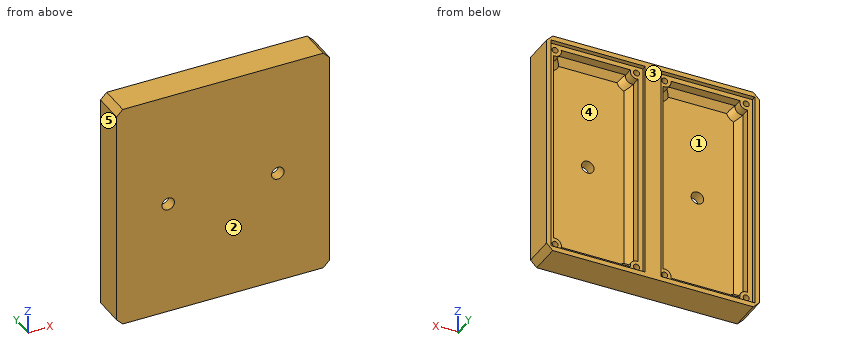
from build123d import *

# Parameters (mm, degrees)
SKETCH2_W           = 68
SKETCH2_H           = 73
SKETCH2_W_2         = 30
SKETCH2_H_2         = 70
BOSS_EXTRUDE1_DEPTH = 10
SKETCH2_3_W         = 30
SKETCH2_3_H         = 70
CUT_EXTRUDE2_DEPTH  = 1.5
SKETCH3_W           = 27
SKETCH3_H           = 67
CUT_EXTRUDE3_DEPTH  = 5
SKETCH4_R           = 2
BOSS_EXTRUDE2_DEPTH = 5
CUT_EXTRUDE4_START  = -5
SKETCH5_R           = 0.95
CUT_EXTRUDE4_DEPTH  = 5
CHAMFER1_SIZE       = 2
CHAMFER2_SIZE       = 2
SKETCH6_R           = 2
CUT_EXTRUDE5_DEPTH  = 4


with BuildPart() as part:
    # Sketch2 → Boss-Extrude1 (new body)
    # profile 1 of 3: a face of its own
    with BuildSketch(Plane(origin=(0, 0, 0), x_dir=(1, 0, 0), z_dir=(0, 1, 0))):
        Rectangle(SKETCH2_W, SKETCH2_H)
        with Locations((17.5, 0)):
            Rectangle(SKETCH2_W_2, SKETCH2_H_2, mode=Mode.SUBTRACT)
        with Locations((-17.5, 0)):
            Rectangle(SKETCH2_W_2, SKETCH2_H_2, mode=Mode.SUBTRACT)
    # profile 2 of 3: a face of its own
    with BuildSketch(Plane(origin=(0, 0, 0), x_dir=(1, 0, 0), z_dir=(0, 1, 0))):
        with Locations((17.5, 0)):
            Rectangle(SKETCH2_W_2, SKETCH2_H_2)
    # profile 3 of 3: a face of its own
    with BuildSketch(Plane(origin=(0, 0, 0), x_dir=(1, 0, 0), z_dir=(0, 1, 0))):
        with Locations((-17.5, 0)):
            Rectangle(SKETCH2_W_2, SKETCH2_H_2)
    extrude(amount=-BOSS_EXTRUDE1_DEPTH)

    # Sketch2<3> → Cut-Extrude2 (cut)
    with BuildSketch(Plane(origin=(0, 0, 0), x_dir=(1, 0, 0), z_dir=(0, 1, 0))):
        with Locations((-17.5, 0)):
            Rectangle(SKETCH2_3_W, SKETCH2_3_H)
        with Locations((17.5, 0)):
            Rectangle(SKETCH2_3_W, SKETCH2_3_H)
    extrude(amount=-CUT_EXTRUDE2_DEPTH, mode=Mode.SUBTRACT)

    # Sketch3 → Cut-Extrude3 (cut)
    with BuildSketch(Plane(origin=(0, -1.5, 0), x_dir=(1, 0, 0), z_dir=(0, 1, 0))):
        with Locations((-17.5, 0)):
            Rectangle(SKETCH3_W, SKETCH3_H)
        with Locations((17.5, 0)):
            Rectangle(SKETCH3_W, SKETCH3_H)
    extrude(amount=-CUT_EXTRUDE3_DEPTH, mode=Mode.SUBTRACT)

    # Sketch4 → Boss-Extrude2 (add)
    with BuildSketch(Plane(origin=(0, -6.5, 0), x_dir=(1, 0, 0), z_dir=(0, 1, 0))):
        with Locations((-30.5, 33)):
            Circle(SKETCH4_R)
        with Locations((-4.5, 33)):
            Circle(SKETCH4_R)
        with Locations((-4.5, -33)):
            Circle(SKETCH4_R)
        with Locations((-30.5, -33)):
            Circle(SKETCH4_R)
        with Locations((30.5, -33)):
            Circle(SKETCH4_R)
        with Locations((4.5, -33)):
            Circle(SKETCH4_R)
        with Locations((4.5, 33)):
            Circle(SKETCH4_R)
        with Locations((30.5, 33)):
            Circle(SKETCH4_R)
    extrude(amount=BOSS_EXTRUDE2_DEPTH)

    # Sketch5 → Cut-Extrude4 (cut)
    with BuildSketch(Plane(origin=(0, -1.5, 0), x_dir=(1, 0, 0), z_dir=(0, 1, 0)).offset(CUT_EXTRUDE4_START)):
        with Locations(Location((-30.5, 33, 0), (0, 0, 270))):
            Circle(SKETCH5_R)
        with Locations(Location((-4.5, 33, 0), (0, 0, 270))):
            Circle(SKETCH5_R)
        with Locations(Location((-4.5, -33, 0), (0, 0, 270))):
            Circle(SKETCH5_R)
        with Locations(Location((-30.5, -33, 0), (0, 0, 270))):
            Circle(SKETCH5_R)
        with Locations(Location((30.5, -33, 0), (0, 0, 270))):
            Circle(SKETCH5_R)
        with Locations(Location((4.5, -33, 0), (0, 0, 270))):
            Circle(SKETCH5_R)
        with Locations(Location((4.5, 33, 0), (0, 0, 270))):
            Circle(SKETCH5_R)
        with Locations(Location((30.5, 33, 0), (0, 0, 270))):
            Circle(SKETCH5_R)
    extrude(amount=CUT_EXTRUDE4_DEPTH, mode=Mode.SUBTRACT)

    # Chamfer1
    chamfer1_edges = [part.edges().sort_by_distance(p)[0] for p in [
        (-34, -5, 36.5),
        (-34, -5, -36.5),
        (34, -5, -36.5),
        (34, -5, 36.5),
    ]]
    chamfer(chamfer1_edges, length=CHAMFER1_SIZE)

    # Chamfer2
    chamfer2_edges = [part.edges().sort_by_distance(p)[0] for p in [
        (-4, -6.5, 0),
        (-5.914213562, -6.5, 31.585786438),
        (-17.5, -6.5, 33.5),
        (-29.085786438, -6.5, 31.585786438),
        (31, -6.5, 0),
        (29.085786438, -6.5, 31.585786438),
        (17.5, -6.5, 33.5),
        (5.914213562, -6.5, 31.585786438),
        (4, -6.5, 0),
        (5.914213562, -6.5, -31.585786438),
        (17.5, -6.5, -33.5),
        (29.085786438, -6.5, -31.585786438),
        (-31, -6.5, 0),
        (-29.085786438, -6.5, -31.585786438),
        (-17.5, -6.5, -33.5),
        (-5.914213562, -6.5, -31.585786438),
    ]]
    chamfer(chamfer2_edges, length=CHAMFER2_SIZE)

    # Sketch6 → Cut-Extrude5 (cut)
    with BuildSketch(Plane.XZ.offset(10)):
        with Locations(Location((-17.5, 0, 0), (0, 0, 270))):
            Circle(SKETCH6_R)
        with Locations(Location((17.5, 0, 0), (0, 0, 270))):
            Circle(SKETCH6_R)
    extrude(amount=-CUT_EXTRUDE5_DEPTH, mode=Mode.SUBTRACT)


solid = part.part
Verification items for the finished model (mm, model axes). Face numbers are marked on the shaded views. A direction names the side the tool comes from. Round coordinates to 2 decimals unless told otherwise and drop trailing zeros. Loops run counter-clockwise (first coordinate to the right, second up) from the corner with the lowest first, then second, coordinate; pieces in that order, holes last. Notation, with made-up numbers: (-14, 65.5) - (33, 65.5) arc R16 cw to (33, 88.5) - close; hole circle Ø9 at (-37, -21). An arc over 180 degrees is marked (long way). Use a Markdown table: item, result. Add a question column.
1. Section check C-C, the plane z = 13.5. Record the boundary of the cut face in (x, y).
2. Thickness scan on probe 1 along X at (y, z) = (-9.25, 0); probe 2 along X at (y, z) = (-1, 17); probe 3 along X at (y, z) = (-5.25, 33). Record the ranges inside material, lowest first. Write a range as [from, to].
3. Section check B-B, the plane x = -17.5. Record the boundary of the cut face in (y, z), plus the area to 3 significant figures.
4. Release check for a two-part mould opening along X. For the marked faces 3, 4 and 5 record: released by +X, released by -X, zero draft, split by the parting line, or undercut.
5. Access from +Z, -Z, +X, -X, +Y, -Y to the whole of each face (thin tool, end or side, straight path). Record for the marked faces 1 and 2.
6. Section check A-A, the plane z = 0. Give the number of separate pieces and of enclosed holes in the cut face, plus the area to 3 significant figures.
7. Gauge pin test, flat ends, axial feed: pin 1 (1.5 mm diameter, centred on x = -4.5, z = 33, fed in from +Y); pin 2 (15 mm diameter, centred on x = 12, z = 5, fed in from +Y); pin 3 (1 mm diameter, centred on x = 5, z = 33, fed in from +Y). Record the tip position at first contact, or that the pin passes through.
Checks:
| question | item | result |
|---|---|---|
| 1 | outline | (-34, -10) - (34, -10) - (34, 0) - (32.5, 0) - (32.5, -1.5) - (31, -1.5) - (31, -4.5) - (29, -6.5) - (6, -6.5) - (4, -4.5) - (4, -1.5) - (2.5, -1.5) - (2.5, 0) - (-2.5, 0) - (-2.5, -1.5) - (-4, -1.5) - (-4, -4.5) - (-6, -6.5) - (-29, -6.5) - (-31, -4.5) - (-31, -1.5) - (-32.5, -1.5) - (-32.5, 0) - (-34, 0) - close |
| 2 | probe 1 | x = [-34, -19.5], [-15.5, 15.5], [19.5, 34] |
| 2 | probe 2 | x = [-34, -32.5], [-2.5, 2.5], [32.5, 34] |
| 2 | probe 3 | x = [-34, -31.45], [-29.55, -5.45], [-3.55, 3.55], [5.45, 29.55], [31.45, 34] |
| 3 | outline | (-10, -36.5) - (0, -36.5) - (0, -35) - (-1.5, -35) - (-1.5, -33.5) - (-4.5, -33.5) - (-6.5, -31.5) - (-6.5, -2) - (-10, -2) - close; (-10, 2) - (-6.5, 2) - (-6.5, 31.5) - (-4.5, 33.5) - (-1.5, 33.5) - (-1.5, 35) - (0, 35) - (0, 36.5) - (-10, 36.5) - close |
| 3 | area | 280 mm^2 |
| 4 | face 3 | zero draft |
| 4 | face 4 | undercut |
| 4 | face 5 | released by -X |
| 5 | face 1 | +Y |
| 5 | face 2 | +Z, -Z, +X, -X, -Y |
| 6 | separate pieces | 3 |
| 6 | enclosed holes | 0 |
| 6 | area | 300 mm^2 |
| 7 | pin 1 | stops at y = -6.5 |
| 7 | pin 2 | stops at y = -5 |
| 7 | pin 3 | stops at y = -1.5 |
